Geometry: see drawing. Coordinates: mm, zero at the bounding-box minimum. A direction names the side the tool comes from. Give positions to 0.01 mm unless a question says otherwise; leave off trailing zeros. Write each loop counter-clockwise with the first axis right and the second up, starting at its lowest first coordinate (ties: lowest second). Pieces come first, ordered by that corner, then holes. Notation, with made-up numbers: M 13.25,80.25 L 45.25,80.25 A32 cw 45.25,108.25 Z; hole C -35,-20.75 d11. An arc over 180 degrees is marked long. Answer as a JSON object with one key per item and string values. Group by question number.
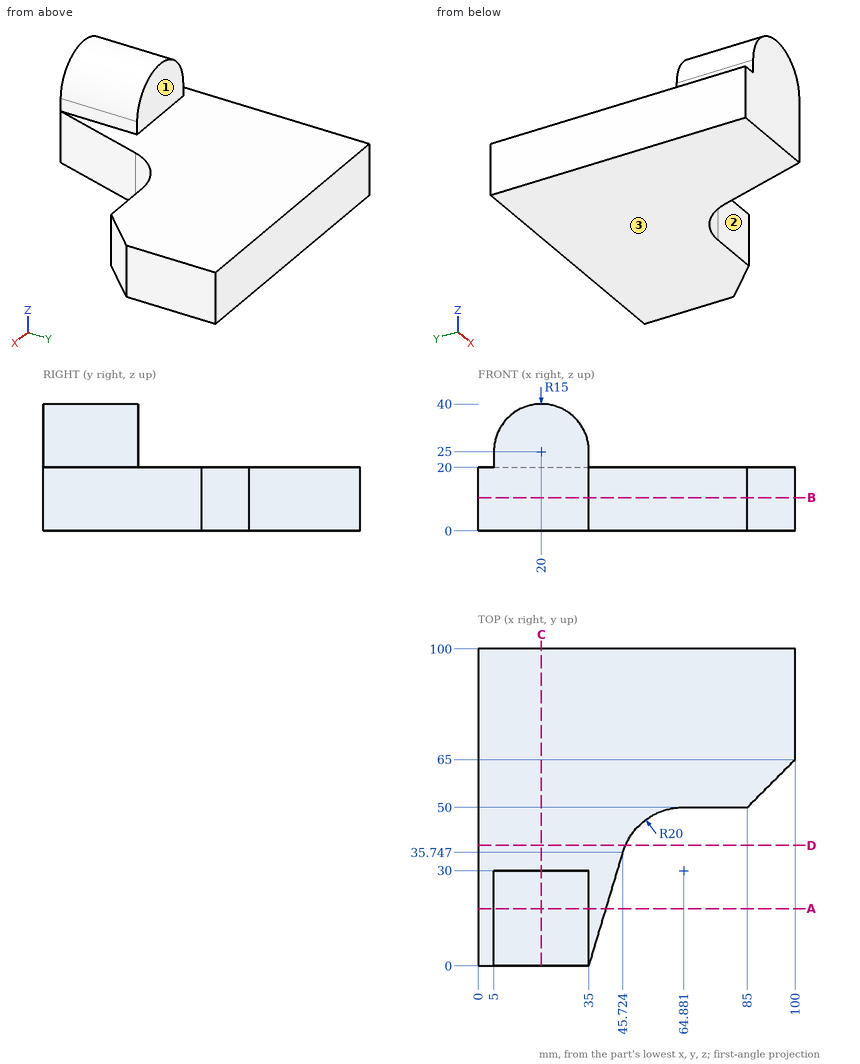
(1) Section A-A, the plane y = 18. Return loops of the section in (x, z), plus the area to 3 significant figures.
(2) Contact query for flat-ended pins moving along their axis: pin 1 Ø2.5 at (y, z) = (16.5, 22.5) entering from +X; pin 2 Ø1 at (y, z) = (23, 9.5) entering from +X; pin 3 Ø2 at (y, z) = (32.5, 28.5) entering from +X; pin 4 Ø5.5 at (y, z) = (10.5, 23.5) entering from -X. Output: stop coordinate, or through.
(3) Section D-D, the plane y = 38. Return loops of the section in (x, z).
(4) Section B-B, the plane z = 10.5. Return loops of the section in (x, y), plus the area to 3 significant figures.
(5) Ray query, L1, parallel to Z at x = 37, y = 60.5; L2, parallel to Y at x = 12, z = 37; L3, parallel to Y at x = 70, z = 16. Return the intervals inside material, ascending. Write a range as [from, to].
(6) Section C-C, the plane x = 20. Return loops of the section in (y, z).
(7) Access query for the marked faces 1, 2 and 3. Directions: +Z, -Z, +X, -X, +Y, -Y. A direction counts if a zero-diameter tool reaches every point of the face in a straight line with its end or side. Return the directions, or none.
Reported:
{
 "1": {"outline": "M 0,0 L 40.4,0 L 40.4,20 L 35,20 L 35,25 A15 ccw 5,25 L 5,20 L 0,20 Z", "area": "1,310 mm2"},
 "2": {"pin 1": "stops at x = 35", "pin 2": "stops at x = 42.05", "pin 3": "passes through", "pin 4": "stops at x = 5"},
 "3": {"outline": "M 0,0 L 46.55,0 L 46.55,20 L 0,20 Z"},
 "4": {"outline": "M 0,0 L 35,0 L 45.72,35.75 A20 cw 64.88,50 L 85,50 L 100,65 L 100,100 L 0,100 Z", "area": "7,050 mm2"},
 "5": {"L1": "z = [0, 20]", "L2": "y = [0, 30]", "L3": "y = [50, 100]"},
 "6": {"outline": "M 0,0 L 100,0 L 100,20 L 30,20 L 30,40 L 0,40 Z"},
 "7": {"face 1": "+Z, +X, -X, +Y", "face 2": "+Z, -Z, +X, -Y", "face 3": "-Z, +X, -X, +Y, -Y"}
}
